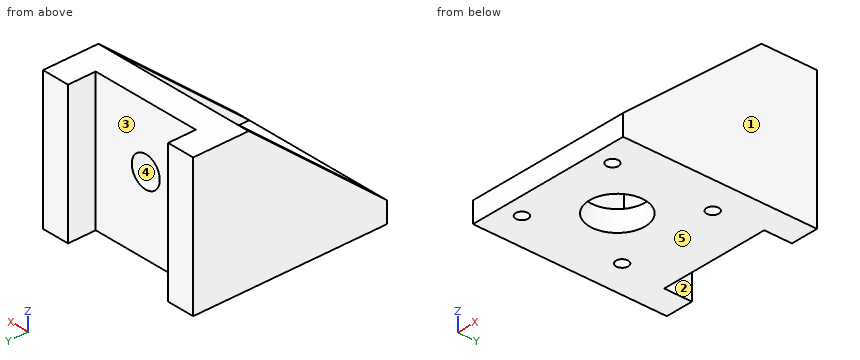
```python
from build123d import *

# Parameters (mm, degrees)
F0_W      = 25.4
F0_H      = 31.75
F1_DEPTH  = 6.35
F2_W      = 6.35
F2_H      = 31.75
F3_DEPTH  = 12.7
F4_W      = 38.1
F4_H      = 4.7625
F5_DEPTH  = 31.75
F7_DEPTH  = 3.175
F9_DEPTH  = 3.175
F10_R     = 3.556
F11_DEPTH = 6.35
F12_R     = 1.4
F12_R_2   = 6.35
F13_DEPTH = 4.7625


with BuildPart() as f1:
    # F0 (on Front) → F1 (new body)
    with BuildSketch(Plane.XZ):
        with Locations((0, 15.875)):
            Rectangle(F0_W, F0_H)
    extrude(amount=F1_DEPTH)

    # F2 (on face) → F3 (join)
    with BuildSketch(Plane.XZ.offset(6.35)):
        with Locations((-15.875, 15.875)):
            Rectangle(F2_W, F2_H)
        with Locations((15.875, 15.875)):
            Rectangle(F2_W, F2_H)
    extrude(amount=-F3_DEPTH)

    # F4 (on face) → F5 (join)
    with BuildSketch(Plane.XZ.offset(6.35)):
        with Locations((0, 2.38125)):
            Rectangle(F4_W, F4_H)
    extrude(amount=F5_DEPTH)

    # F6 (on face) → F7 (join)
    with BuildSketch(Plane(origin=(-19.05, 0, 0), x_dir=(0, -1, 0), z_dir=(-1, 0, 0))):
        Polygon((38.1, 4.7625), (6.35, 31.75), (6.35, 4.7625), align=None)
    extrude(amount=-F7_DEPTH)

    # F8 (on face) → F9 (join)
    with BuildSketch(Plane.YZ.offset(19.05)):
        Polygon((-6.35, 4.7625), (-6.35, 31.75), (-38.1, 4.7625), align=None)
    extrude(amount=-F9_DEPTH)

    # F10 (on Front) → F11 (cut)
    with BuildSketch(Plane.XZ):
        with Locations((0, 17.508461)):
            Circle(F10_R)
    extrude(amount=F11_DEPTH, mode=Mode.SUBTRACT)

    # F12 (on face) → F13 (cut, through all)
    with BuildSketch(Plane.XY.offset(4.7625)):
        with Locations((11.4935, -33.7185)):
            Circle(F12_R)
        with Locations((-11.4935, -33.7185)):
            Circle(F12_R)
        with Locations((11.4935, -10.7315)):
            Circle(F12_R)
        with Locations((-11.4935, -10.7315)):
            Circle(F12_R)
        with Locations((0, -22.225)):
            Circle(F12_R_2)
    extrude(amount=-F13_DEPTH, mode=Mode.SUBTRACT)


solid = f1.part
```
Geometry: final body of the model. Coordinates: model frame, mm. Face numbers are marked on the shaded views. A direction names the side the tool comes from. Round coordinates to 2 decimals unless told otherwise and drop trailing zeros. Write each loop counter-clockwise with the first axis right and the second up, starting at its lowest first coordinate (ties: lowest second). Pieces come first, ordered by that corner, then holes.
Item 1: Section query B-B (x = -5.5). Return loops of the section in (y, z), plus the area to 3 significant figures.
Item 2: Section query D-D (z = 24.5). Return loops of the section in (x, y) (3 decimals), plus the area to 3 significant figures.
Item 3: Mould query, pull axis Z, two halves, no side actions, for the marked faces 3, 4 and 5. Classes: +Z half, -Z half, draft (parallel to the pull), parting line (faces both ways), or undercut.
Item 4: Set-up query: the marked faces 1 and 2. Return all of +Z, -Z, +X, -X, +Y, -Y with unobstructed straight access to the full face (end or side cutting, diameter ignored); none if empty.
Item 5: Material intervals for L1, parallel to Z at x = 0, y = -4; L2, parallel to X at y = -10, z = 14 (3 decimals); L3, parallel to X at y = 3, z = 6, sorted ascending.
Item 6: Pin query (flat end, axial travel): P1, Ø6, axis at x = -9.5, z = 15.5, coming from the +Y side; P2, Ø1.7, axis at x = 11.49, y = -33.72, coming from the +Z side; P3, Ø3.5, axis at x = -11.49, y = -10.73, coming from the +Z side; P4, Ø2, axis at x = -14, z = 10, coming from the -Y side. Return the tip coordinate at first contact, or that it passes through.
Item 7: Section query A-A (x = 0). Give the number of separate pieces and of enclosed holes in the cut face, plus the area to 3 significant figures.
Completed:
1. outline: (-38.1, 0) - (-25.4, 0) - (-25.4, 4.76) - (-38.1, 4.76) - close; (-19.05, 0) - (0, 0) - (0, 31.75) - (-6.35, 31.75) - (-6.35, 4.76) - (-19.05, 4.76) - close
1. area: 323 mm2
2. outline: (-19.05, -14.879) - (-15.875, -14.879) - (-15.875, -6.35) - (15.875, -6.35) - (15.875, -14.879) - (19.05, -14.879) - (19.05, 6.35) - (12.7, 6.35) - (12.7, 0) - (-12.7, 0) - (-12.7, 6.35) - (-19.05, 6.35) - close
2. area: 377 mm2
3. face 3: draft
3. face 4: undercut
3. face 5: -Z half
4. face 1: +Z, -Z, +X, +Y, -Y
4. face 2: +Z, -Z, +Y
5. L1: z = 0 to 13.95, 21.06 to 31.75
5. L2: x = -19.05 to -15.875, 15.875 to 19.05
5. L3: x = -19.05 to -12.7, 12.7 to 19.05
6. P1: stops at y = 0
6. P2: passes through
6. P3: stops at z = 4.76
6. P4: stops at y = -6.35
7. separate pieces: 3
7. enclosed holes: 0
7. area: 247 mm2
